```python
from build123d import *

# Parameters (mm, degrees)
IZIM1_R                     = 350
Y_KSEKLIK_EKSTR_ZYON1_DEPTH = 5


with BuildPart() as part:
    # Çizim1 → Yükseklik-Ekstrüzyon1 (new body)
    with BuildSketch(Plane(origin=(0, 0, 0), x_dir=(1, 0, 0), z_dir=(0, 1, 0))):
        with Locations(Location((0, 0, 0), (0, 0, 270))):
            Circle(IZIM1_R)
        with BuildLine():
            Line((82.608627247, 56.354367216), (169.455080757, 106.495190528))
            Line((169.455080757, 106.495190528), (176.955080757, 93.504809472))
            Line((176.955080757, 93.504809472), (90.108627247, 43.36398616))
            ThreePointArc((90.108627247, 43.36398616), (100, 0), (90.108627247, -43.36398616))
            Line((90.108627247, -43.36398616), (176.955080757, -93.504809472))
            Line((176.955080757, -93.504809472), (169.455080757, -106.495190528))
            Line((169.455080757, -106.495190528), (82.608627247, -56.354367216))
            ThreePointArc((82.608627247, -56.354367216), (50, -86.602540378), (7.5, -99.718353376))
            Line((7.5, -99.718353376), (7.5, -200))
            Line((7.5, -200), (-7.5, -200))
            Line((-7.5, -200), (-7.5, -99.718353376))
            ThreePointArc((-7.5, -99.718353376), (-50, -86.602540378), (-82.608627247, -56.354367216))
            Line((-82.608627247, -56.354367216), (-169.455080757, -106.495190528))
            Line((-169.455080757, -106.495190528), (-176.955080757, -93.504809472))
            Line((-176.955080757, -93.504809472), (-90.108627247, -43.36398616))
            ThreePointArc((-90.108627247, -43.36398616), (-100, 0), (-90.108627247, 43.36398616))
            Line((-90.108627247, 43.36398616), (-176.955080757, 93.504809472))
            Line((-176.955080757, 93.504809472), (-169.455080757, 106.495190528))
            Line((-169.455080757, 106.495190528), (-82.608627247, 56.354367216))
            ThreePointArc((-82.608627247, 56.354367216), (-50, 86.602540378), (-7.5, 99.718353376))
            Line((-7.5, 99.718353376), (-7.5, 200))
            Line((-7.5, 200), (7.5, 200))
            Line((7.5, 200), (7.5, 99.718353376))
            ThreePointArc((7.5, 99.718353376), (50, 86.602540378), (82.608627247, 56.354367216))
        make_face(mode=Mode.SUBTRACT)
        with BuildLine():
            Line((246.056268189, 111.158953237), (289.538139145, 136.263223139))
            ThreePointArc((289.538139145, 136.263223139), (318.878995434, -26.761656733), (262.776482412, -182.615772295))
            Line((262.776482412, -182.615772295), (219.294611456, -157.511502394))
            ThreePointArc((219.294611456, -157.511502394), (268.670455631, -26.761656733), (246.056268189, 111.158953237))
        make_face(mode=Mode.SUBTRACT)
    extrude(amount=Y_KSEKLIK_EKSTR_ZYON1_DEPTH)


solid = part.part
```
The model under review builds one solid part; all positions refer to its coordinate system, in mm. A direction names the side the tool comes from. Give positions to 0.01 mm unless a question says otherwise; leave off trailing zeros. Loops run counter-clockwise (first coordinate to the right, second up) from the corner with the lowest first, then second, coordinate; pieces in that order, holes last. Notation, with made-up numbers: (67, -28.5) -> (107, -28.5) arc R27 ccw to (107, -4.5) -> close; hole circle Ø5 at (52.25, 80). An arc over 180 degrees is marked (long way). Use CSV: the item, a comma, the result in double quotes.
1. To check wall thickness, follow probe 1 along Z at (x, y) = (-4, 2.1); probe 2 along Z at (x, y) = (116, 2.95); probe 3 along X at (y, z) = (2.65, -100). State the ranges of each line that lie inside material, in increasing order. Write a range as from..to.
Result:
probe 1,"z = -349.98..-200, 200..349.98"
probe 2,"z = -330.22..-75.63, -58.31..58.31, 75.63..330.22"
probe 3,"x = -335.41..-173.21, -158.21..-7.5, 7.5..158.21, 173.21..250.8, 303.97..335.41"
2. Consider section A-A, the plane z = 0. Write out the cut boundary in (x, y), then the cut area to 3 significant figures.
Result:
outline,"(-350, 0) -> (-100, 0) -> (-100, 5) -> (-350, 5) -> close; (100, 0) -> (270, 0) -> (270, 5) -> (100, 5) -> close; (320, 0) -> (350, 0) -> (350, 5) -> (320, 5) -> close"
area,"2,250 mm²"
3. The part is to be moulded in two halves that separate along Z. For faces 3 (the face through (-73, 5, 73)), 4 (the face through (-132.92, 2.46, -68.08)), 5 (the face through (319.067, 2.465, 24.423)), 6 (the face through (347.022, 2.465, -45.563)), say which applies: +Z half, -Z half, draft (parallel to the pull), parting line (faces both ways), or undercut.
Result:
face 3,"draft"
face 4,"undercut"
face 5,"undercut"
face 6,"parting line"
4. Consider section D-D, the plane x = -160. Write out the cut boundary in (y, z), then the cut area to 3 significant figures.
Result:
outline,"(0, -311.29) -> (5, -311.29) -> (5, -101.04) -> (0, -101.04) -> close; (0, -83.72) -> (5, -83.72) -> (5, 83.72) -> (0, 83.72) -> close; (0, 101.04) -> (5, 101.04) -> (5, 311.29) -> (0, 311.29) -> close"
area,"2,940 mm²"
5. Consider section B-B, the plane x = 302. Write out the cut boundary in (y, z), then the cut area to 3 significant figures.
Result:
outline,"(0, -176.91) -> (5, -176.91) -> (5, -105.81) -> (0, -105.81) -> close; (0, 105.81) -> (5, 105.81) -> (5, 176.91) -> (0, 176.91) -> close"
area,"711 mm²"
6. Consider section C-C, the plane y = 3.2. Count the separate pieces of the cut face and the enclosed holes in it, then the cut area to 3 significant figures.
Result:
separate pieces,"1"
enclosed holes,"2"
area,"329,000 mm²"
7. Machinability: for faces 1 (the face through (-73, 0, 73)), 2 (the face through (125.42, 2.46, -81.07)), which of the approach directions +Z, -Z, +X, -X, +Y, -Y give a long, thin tool a straight path to every point of the face, cutting with its end or side? Answer none if there is none.
Result:
face 1,"+Z, -Z, +X, -X, -Y"
face 2,"+Y, -Y"
8. For P1, Ø4, axis at x = -45.5, z = -95, coming from the -Y side; P2, Ø2.5, axis at y = 2, z = -173.5, coming from the -X side; P3, Ø1, axis at x = -240.5, y = 0.5, coming from the +Z side; P4, Ø1.5, axis at y = 1.5, z = -170.5, coming from the +X side, all flat-tipped, find the tip position at first contact; note any pin that passes through.
Result:
P1,"stops at y = 0"
P2,"stops at x = -304.68"
P3,"stops at z = 254.75"
P4,"stops at x = 306.08"
